from build123d import *

# Parameters (mm, degrees)
BOSS_EXTRUDE2_DEPTH = 20.32
FILLET1_R           = 25.4
FILLET2_R           = 25.4
FILLET3_R           = 25.4
FILLET4_R           = 25.4
CUT_EXTRUDE1_DEPTH  = 20.32
FILLET5_R           = 2.54


with BuildPart() as part:
    # Sketch1 → Boss-Extrude2 (new body)
    with BuildSketch(Plane.XY):
        with BuildLine():
            add(Edge.make_bspline(
                [(-131.195332136, 32.798833034), (2.154667864, 58.198833034), (135.504667864, 32.798833034)],
                knots=[0, 0, 0, 1, 1, 1], degree=2))
            add(Edge.make_bspline(
                [(135.504667864, 32.798833034), (186.304667864, -43.401166966), (135.504667864, -119.601166966)],
                knots=[0, 0, 0, 1, 1, 1], degree=2))
            add(Edge.make_bspline(
                [(-131.195332136, -119.601166966), (2.154667864, -94.201166966), (135.504667864, -119.601166966)],
                knots=[0, 0, 0, 1, 1, 1], degree=2))
            add(Edge.make_bspline(
                [(-131.195332136, 32.798833034), (-181.995332136, -43.401166966), (-131.195332136, -119.601166966)],
                knots=[0, 0, 0, 1, 1, 1], degree=2))
        make_face()
    extrude(amount=BOSS_EXTRUDE2_DEPTH)

    # Fillet1
    fillet1_edges = [part.edges().sort_by_distance(p)[0] for p in [
        (135.504667864, -119.601166966, 10.16),
    ]]
    fillet(fillet1_edges, radius=FILLET1_R)

    # Fillet2
    fillet2_edges = [part.edges().sort_by_distance(p)[0] for p in [
        (-131.195332136, -119.601166966, 10.16),
    ]]
    fillet(fillet2_edges, radius=FILLET2_R)

    # Fillet3
    fillet3_edges = [part.edges().sort_by_distance(p)[0] for p in [
        (135.504667864, 32.798833034, 10.16),
    ]]
    fillet(fillet3_edges, radius=FILLET3_R)

    # Fillet4
    fillet4_edges = [part.edges().sort_by_distance(p)[0] for p in [
        (-131.195332136, 32.798833034, 10.16),
    ]]
    fillet(fillet4_edges, radius=FILLET4_R)

    # Sketch2 → Cut-Extrude1 (cut)
    with BuildSketch(Plane.XY.offset(20.32)):
        with BuildLine():
            Line((-118.089671205, 20.173896233), (-70.845671205, 20.173896233))
            Line((-70.845671205, 20.173896233), (-70.845671205, -87.716522063))
            Line((-70.845671205, -87.716522063), (-118.089671205, -87.716522063))
            ThreePointArc((-118.089671205, -87.716522063), (-127.069927326, -83.996778184), (-130.789671205, -75.016522063))
            Line((-130.789671205, -75.016522063), (-130.789671205, 7.473896233))
            ThreePointArc((-130.789671205, 7.473896233), (-127.069927326, 16.454152354), (-118.089671205, 20.173896233))
        make_face()
        with BuildLine():
            Line((135.099006932, 7.473896233), (135.099006932, -75.016522063))
            ThreePointArc((135.099006932, -75.016522063), (131.379263053, -83.996778184), (122.399006932, -87.716522063))
            Line((122.399006932, -87.716522063), (75.155006932, -87.716522063))
            Line((75.155006932, -87.716522063), (75.155006932, 20.173896233))
            Line((75.155006932, 20.173896233), (122.399006932, 20.173896233))
            ThreePointArc((122.399006932, 20.173896233), (131.379263053, 16.454152354), (135.099006932, 7.473896233))
        make_face()
    extrude(amount=-CUT_EXTRUDE1_DEPTH, mode=Mode.SUBTRACT)

    # Fillet5
    fillet5_edges = [part.edges().sort_by_distance(p)[0] for p in [
        (-127.069927326, 16.454152354, 0),
        (-94.467671205, 20.173896233, 20.32),
        (-70.845671205, -33.771312915, 20.32),
        (-94.467671205, -87.716522063, 0),
        (-127.069927326, -83.996778184, 0),
        (-130.789671205, -33.771312915, 0),
        (-94.467671205, 20.173896233, 0),
        (-70.845671205, -33.771312915, 0),
        (-127.069927326, 16.454152354, 20.32),
        (-130.789671205, -33.771312915, 20.32),
        (-127.069927326, -83.996778184, 20.32),
        (-94.467671205, -87.716522063, 20.32),
        (98.777006932, 20.173896233, 20.32),
        (131.379263053, 16.454152354, 20.32),
        (135.099006932, -33.771312915, 20.32),
        (131.379263053, -83.996778184, 0),
        (98.777006932, -87.716522063, 0),
        (75.155006932, -33.771312915, 0),
        (98.777006932, 20.173896233, 0),
        (131.379263053, 16.454152354, 0),
        (135.099006932, -33.771312915, 0),
        (75.155006932, -33.771312915, 20.32),
        (98.777006932, -87.716522063, 20.32),
        (131.379263053, -83.996778184, 20.32),
    ]]
    fillet(fillet5_edges, radius=FILLET5_R)


solid = part.part
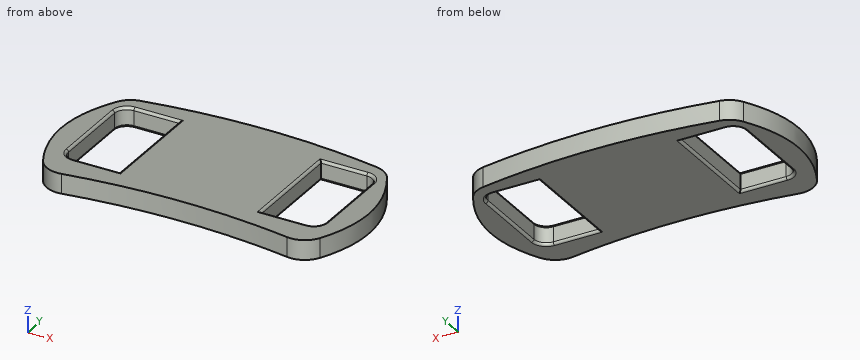
Input: part model. Units: mm. Frame: model coordinates. Give positions to 0.01 mm unless a question says otherwise; leave off trailing zeros. Use CSV: the item, a comma, the result in double quotes. Start each with the question number.
Item 1: Contact query for flat-ended pins moving along their axis: P1, Ø4.5, axis at y = -33.5, z = 13, coming from the -X side; P2, Ø7.5, axis at y = -13, z = 6.5, coming from the +X side; P3, Ø3, axis at y = 11, z = 7.5, coming from the +X side. Output: stop coordinate, or through.
Item 2: Section A-A on z = 13.75. State how many separate pieces and enclosed holes the cut face has, then the cut area to 3 significant figures.
Item 3: Line query: line 1 (X direction, y = -42, z = 14.5) (3 decimals); line 2 (X direction, y = -53.5, z = 8) (3 decimals); line 3 (Y direction, x = -98, z = 15.5). Output: solid intervals per line, ascending.
Ans:
1,P1,"stops at x = -156.34"
1,P2,"stops at x = 157.8"
1,P3,"stops at x = 148.66"
2,separate pieces,"1"
2,enclosed holes,"2"
2,area,"32,900 mm2"
3,line 1,"x = -156.587 to -130.79, -70.846 to 75.155, 135.099 to 160.896"
3,line 2,"x = -156.149 to -130.79, -70.846 to 75.155, 135.099 to 160.459"
3,line 3,"y = -114.07 to -87.72, 20.17 to 38.33"
